```python
from build123d import *

# Parameters (mm, degrees)
F0_W     = 50
F0_H     = 6
F2_DEPTH = 130
F0_H_2   = 100
F0_H_3   = 74
F3_DEPTH = 6
F4_R     = 20
F5_R     = 10
F7_DEPTH = 6
F9_DEPTH = 31


# Not quite as in the source:
# - a feature names something its author has since deleted; it is built from what else it names


with BuildPart() as f2:
    # F0 (on Front) → F2 (new body)
    with BuildSketch(Plane.XZ):
        with Locations((-5, -147)):
            Rectangle(F0_W, F0_H)
    extrude(amount=F2_DEPTH)

    # F0 (on Front) → F3 (join)
    with BuildSketch(Plane.XZ):
        with Locations((-5, -20)):
            Rectangle(F0_W, F0_H_2)
        with Locations((-5, -107)):
            Rectangle(F0_W, F0_H_3)
        with Locations((-5, -147)):
            Rectangle(F0_W, F0_H)
    extrude(amount=F3_DEPTH)

    # F4
    f4_edges = [f2.edges().sort_by_distance(p)[0] for p in [
        (-5, 0, -150),
    ]]
    fillet(f4_edges, radius=F4_R)

    # F5
    f5_edges = [f2.edges().sort_by_distance(p)[0] for p in [
        (-5, -6, -144),
    ]]
    fillet(f5_edges, radius=F5_R)

    # F6 (on face) → F7 (join)
    with BuildSketch(Plane.XY.offset(-144)):
        with BuildLine():
            ThreePointArc((-30, -84.6159367699), (-69.042085877, -79.9604861418), (-107.415399673, -71.3903940482))
            ThreePointArc((-107.415399673, -71.3903940482), (-5.4112498239, -247.9992833605), (97.8214378821, -72.1056832508))
            ThreePointArc((97.8214378821, -72.1056832508), (59.233233327, -80.4336085853), (20, -84.8105109003))
            Line((20, -84.8105109003), (20, -130))
            Line((20, -130), (-30, -130))
            Line((-30, -130), (-30, -84.6159367699))
        make_face()
    extrude(amount=-F7_DEPTH)

    # F8 (on face) → F9 (cut)
    with BuildSketch(Plane.XY.offset(-144)):
        with BuildLine():
            Line((-81.2895118016, -99.9348974879), (-86.618032779, -97.1768430661))
            ThreePointArc((-86.618032779, -97.1768430661), (-77.8915033239, -179.2513111401), (-5, -217.9708071228))
            ThreePointArc((-5, -217.9708071228), (67.8915033239, -179.2513111401), (76.618032779, -97.1768430661))
            Line((76.618032779, -97.1768430661), (71.2895118016, -99.9348974879))
            ThreePointArc((71.2895118016, -99.9348974879), (62.7839892821, -176.1446724661), (-5, -212))
            ThreePointArc((-5, -212), (-72.7839892821, -176.1446724661), (-81.2895118016, -99.9348974879))
        make_face()
    extrude(amount=-F9_DEPTH, mode=Mode.SUBTRACT)


solid = f2.part
```
CAD build for the part. Positions are in the model's coordinates, mm. A direction names the side the tool comes from. Give positions to 0.01 mm unless a question says otherwise; leave off trailing zeros. Loops run counter-clockwise (first coordinate to the right, second up) from the corner with the lowest first, then second, coordinate; pieces in that order, holes last. Notation, with made-up numbers: (-11.5, 86) - (30.5, 86) arc R29 ccw to (30.5, 115) - close; hole circle Ø9 at (22, -24). An arc over 180 degrees is marked (long way). Put each result on its own line as item: value.
Q1. Slice it at A-A (y = -130). Give the cut face in (x, z), plus the area to 3 significant figures.
Filled in:
outline: (-123, -150) - (-92.97, -150) - (-92.97, -144) - (-123, -144) - close; (-87, -150) - (77, -150) - (77, -144) - (-87, -144) - close; (82.97, -150) - (113, -150) - (113, -144) - (82.97, -144) - close
area: 1,340 mm²
Q2. Tool access for faces 4 (the face through (59.779, -80.344, -146.958)), 5 (the face through (-5, 0, -49)), 6 (the face through (-7, -156, -144)): list every direction of +Z, -Z, +X, -X, +Y, -Y with a clear straight run to the whole face (end or side of a thin tool).
Filled in:
face 4: +Z, -Z, +Y
face 5: +Z, -Z, +X, -X, +Y
face 6: +Z, +X, -X, -Y
Q3. Slice it at B-B (x = 25). Give the cut face in (y, z).
Filled in:
outline: (-244.12, -150) - (-212.7, -150) - (-212.7, -144) - (-244.12, -144) - close; (-206.32, -150) - (-84.48, -150) - (-84.48, -144) - (-206.32, -144) - close
Q4. Mould opens along X. For faces 1 (the face through (-7, -132, -150)), 2 (the face through (-68.499, -80.053, -146.958)), 3 (the face through (-8.858, -247.937, -146.958)) say: pulls with the +X half, pulls with the -X half, needs draft (parallel to the pull), parting line crosses it, or undercut.
Filled in:
face 1: needs draft
face 2: undercut
face 3: parting line crosses it
Q5. Slice it at C-C (y = -169.5). Give the cut face in (x, z).
Filled in:
outline: (-116.19, -150) - (-83.6, -150) - (-83.6, -144) - (-116.19, -144) - close; (-76.86, -150) - (66.86, -150) - (66.86, -144) - (-76.86, -144) - close; (73.6, -150) - (106.19, -150) - (106.19, -144) - (73.6, -144) - close
Q6. Slice it at D-D (z = -37). Give the cut face in (x, y), plus the area to 3 significant figures.
Filled in:
outline: (-30, -6) - (20, -6) - (20, 0) - (-30, 0) - close
area: 300 mm²
Q7. Probe line 1 along Z through (x, y) = (42.5, -183); line 2 along Y through (x, z) = (-11, -115); line 3 along Y through (x, z) = (-1.5, -138). List the from-to ranges inside material, lowest first.
Filled in:
line 1: z = -150 to -144
line 2: y = -6 to 0
line 3: y = -6.83 to -1.67
Q8. Flat gauge pin, fed straight in: pin 1 (12 mm diameter, centred on x = -30, z = -0.5, fed in from -Y). Where does the tip first touch, or does it go through?
Filled in:
pin 1: stops at y = -6
